For this review, use the dimensioned drawing (mm, ordinates from the lowest corner) and the shaded views. A direction names the side the tool comes from. Coordinates: 2 decimals unless noted, no trailing zeros. Loops run counter-clockwise (first coordinate to the right, second up) from the corner with the lowest first, then second, coordinate; pieces in that order, holes last. Notation, with made-up numbers: (-5.5, -3) - (15.5, -3) arc R21 ccw to (15.5, 8) - close; hole circle Ø9 at (0, -11.75). An arc over 180 degrees is marked (long way). Answer in a Markdown table with one row per item. Add a question column.
(1) We need section D-D on z = 11.5. Write out the cut boundary in (x, y), plus the area to 3 significant figures.
(2) For P1, Ø1, axis at x = 48, y = 33.5, coming from the -Z side; P2, Ø4.5, axis at x = 46.99, y = 16.25, coming from the +Z side (1 decimal); P3, Ø1.5, axis at x = 35.5, z = 14, coming from the -Y side, all flat-tipped, find the tip position at first contact; note any pin that passes through.
(3) For line 1 along Y through (x, z) = (27.5, 8.5); line 2 along X through (y, z) = (27, 4.75); line 3 along Y through (x, z) = (27.5, 17.5), list the stretches that pass through material, from the lowest coordinate up.
(4) Mouldability with a two-part tool opening along X and no side actions: class the marked faces 3, 4 and 5 as +X half, -X half, draft (parallel to the pull), parting line (faces both ways), or undercut.
(5) We need section B-B on y = 27.5. Write out the cut boundary in (x, z).
(6) We need section A-A on x = 27.5. Write out the cut boundary in (y, z).
(7) Machinability: for the marked faces 1 and 2, which of the approach directions +Z, -Z, +X, -X, +Y, -Y give a long, thin tool a straight path to every point of the face, cutting with its end or side? Answer none if there is none.
(8) We need section C-C on y = 16.25. Give the number of separate pieces and of enclosed holes in the cut face, plus the area to 3 significant figures.
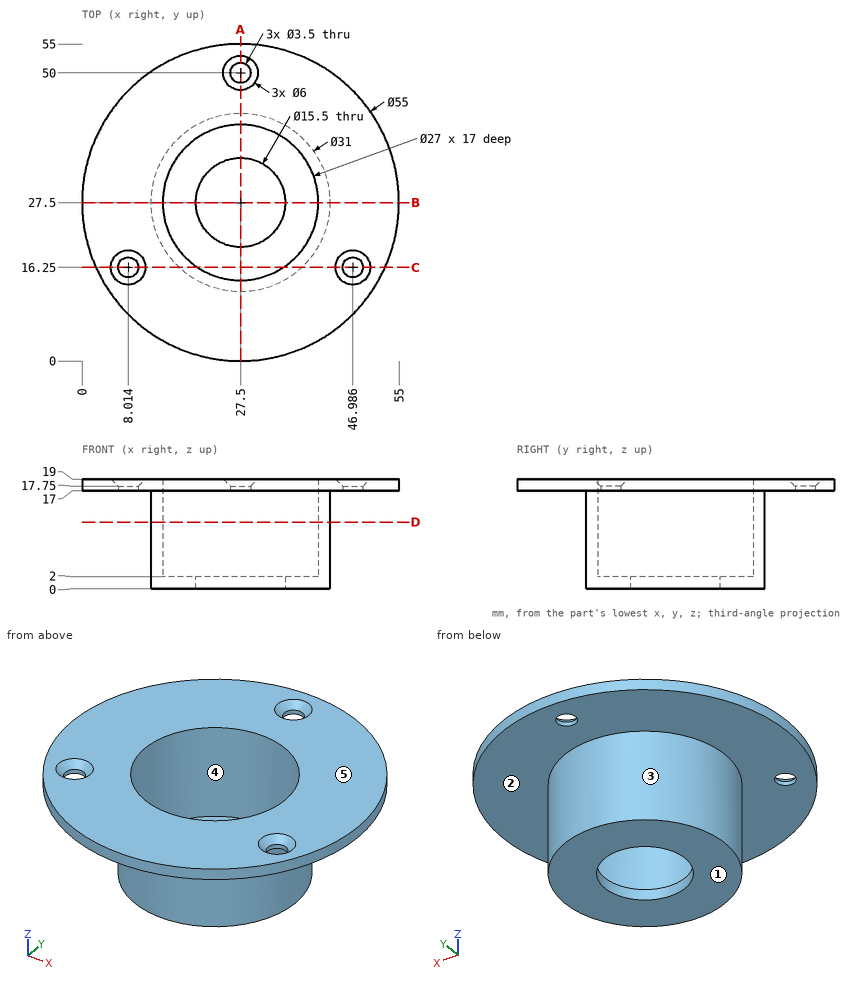
Outcome:
| question | item | result |
|---|---|---|
| 1 | outline | circle Ø31 at (27.5, 27.5); hole circle Ø27 at (27.5, 27.5) |
| 1 | area | 182 mm² |
| 2 | P1 | z = 17 |
| 2 | P2 | z = 18.3 |
| 2 | P3 | y = 13.8 |
| 3 | line 1 | 12 to 14, 41 to 43 |
| 3 | line 2 | 12.01 to 14.01, 40.99 to 42.99 |
| 3 | line 3 | 0 to 14, 41 to 48.25, 51.75 to 55 |
| 4 | face 3 | parting line |
| 4 | face 4 | undercut |
| 4 | face 5 | draft |
| 5 | outline | (0, 17) - (12, 17) - (12, 0) - (19.75, 0) - (19.75, 2) - (14, 2) - (14, 19) - (0, 19) - close; (35.25, 0) - (43, 0) - (43, 17) - (55, 17) - (55, 19) - (41, 19) - (41, 2) - (35.25, 2) - close |
| 6 | outline | (0, 17) - (12, 17) - (12, 0) - (19.75, 0) - (19.75, 2) - (14, 2) - (14, 19) - (0, 19) - close; (35.25, 0) - (43, 0) - (43, 17) - (48.25, 17) - (48.25, 17.75) - (47, 19) - (41, 19) - (41, 2) - (35.25, 2) - close; (51.75, 17) - (55, 17) - (55, 19) - (53, 19) - (51.75, 17.75) - close |
| 7 | face 1 | -Z, +X, -X, +Y, -Y |
| 7 | face 2 | -Z |
| 8 | separate pieces | 3 |
| 8 | enclosed holes | 0 |
| 8 | area | 192 mm² |
